Autodesk Inventor part; units mm, degrees
ref_plane "YZ Plane" through (0, 0, 0) normal (1, 0, 0) x (0, 1, 0)
ref_plane "XZ Plane" through (0, 0, 0) normal (0, 1, 0) x (-1, 0, 0)
ref_plane "XY Plane" through (0, 0, 0) normal (0, 0, 1) x (1, 0, 0)
sketch "スケッチ1" plane through (0, 0, 0) normal (0, 0, 1) x (1, 0, 0)
  circle A0 centre (0, 0) radius 1.3
  dimension "d0" = 2.6
extrude "押し出し1" add sketch "スケッチ1" against normal blind 6
sketch "スケッチ2" plane through (0, 0, 0) normal (0, 0, 1) x (1, 0, 0)
  circle A0 centre (0, 0) radius 2.25
  dimension "d3" = 4.5
extrude "押し出し2" add sketch "スケッチ2" along normal blind 1.7
fillet "フィレット1" radius 1.7 1 edges at (-2.25, 0, 1.7)
thread "ねじ1"
properties part number "ネジ鍋m2.6,06" material "鋼、高強度、低合金"
Check sheet for the modelled part. Datum: model origin and axes. Units: mm. A direction names the side the tool comes from. Round coordinates to 2 decimals unless told otherwise and drop trailing zeros. Loops run counter-clockwise (first coordinate to the right, second up) from the corner with the lowest first, then second, coordinate; pieces in that order, holes last. Notation, with made-up numbers: M 58.25,-40 L 98.25,-40 A12 ccw 98.25,-32 Z; hole C -8,35 d11. An arc over 180 degrees is marked long. One line per item, written item: value.
(1) Access from +Z, -Z, +X, -X, +Y, -Y to the whole of each face (thin tool, end or side, straight path). Record for faces 1 (the face through (0, -1.5, 0)), 2 (the face through (0, 0, -6)).
Computed values:
face 1: -Z
face 2: -Z, +X, -X, +Y, -Y
(2) Depth check by flat-ended pin: pin 1 Ø2 at (y, z) = (-1.5, 0) entering from +X; pin 2 Ø2 at (x, z) = (1, -4) entering from +Y; pin 3 Ø2 at (y, z) = (-1.5, -3.5) entering from +X. Enter the tip coordinate at first touch or a pass-through.
Computed values:
pin 1: stops at x = 2.19
pin 2: stops at y = 1.3
pin 3: stops at x = 1.2
(3) Sectioned sample at A-A, the plane z = -4. Record the cut outline in (x, y).
Computed values:
outline: C 0,0 d2.6
(4) Thickness scan on line 1 (Z direction, x = 0.95, y = -0.35); line 2 (Z direction, x = 1.4, y = 0.2); line 3 (X direction, y = 0.7, z = -3.75). Record the ranges inside material, lowest first.
Computed values:
line 1: z = -6 to 1.64
line 2: z = 0 to 1.46
line 3: x = -1.1 to 1.1
